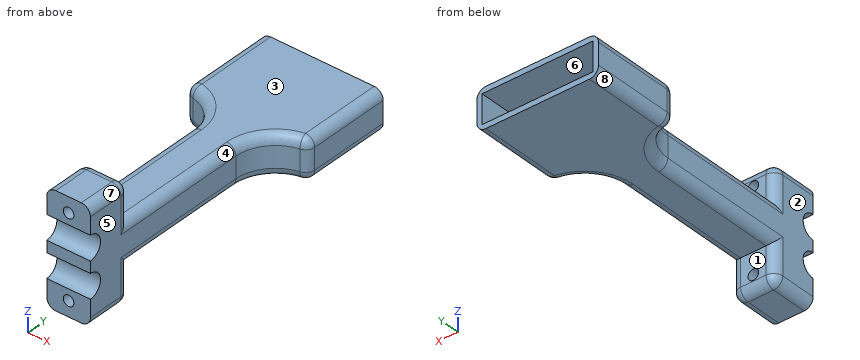
from build123d import *

# Parameters (mm, degrees)
RESSALTO_EXTRUS_O1_DEPTH = 6.5
FILETE1_R                = 3
FILETE2_R                = 3
FILETE3_R                = 13
ESBO_O4_W                = 36.5
ESBO_O4_H                = 9.5
CORTE_EXTRUS_O1_DEPTH    = 25
ESBO_O11_W               = 14.347963754
ESBO_O11_H               = 15
RESSALTO_EXTRUS_O5_DEPTH = 12
ESBO_O17_W               = 14.347963754
ESBO_O17_H               = 15
RESSALTO_EXTRUS_O6_DEPTH = 12
ESBO_O18_R               = 1.75
CORTE_EXTRUS_O5_DEPTH    = 25
ESBO_O19_R               = 3.96875
CORTE_EXTRUS_O6_DEPTH    = 25
FILETE14_R               = 3


with BuildPart() as part:
    # Esboço2 → Ressalto-extrusão1 (new body, symmetric)
    with BuildSketch(Plane.XY):
        Polygon((-20, 50), (20, 50), (20, 20), (7.173981877, 20), (7.173981877, -50), (-7.173981877, -50), (-7.173981877, 20), (-20, 20), align=None)
    extrude(amount=RESSALTO_EXTRUS_O1_DEPTH, both=True)

    # Filete1
    filete1_edges = [part.edges().sort_by_distance(p)[0] for p in [
        (-20, 20, 0),
    ]]
    fillet(filete1_edges, radius=FILETE1_R)

    # Filete2
    filete2_edges = [part.edges().sort_by_distance(p)[0] for p in [
        (20, 20, 0),
    ]]
    fillet(filete2_edges, radius=FILETE2_R)

    # Filete3
    filete3_edges = [part.edges().sort_by_distance(p)[0] for p in [
        (-7.173981877, 20, 0),
        (7.173981877, 20, 0),
    ]]
    fillet(filete3_edges, radius=FILETE3_R)

    # Esboço4 → Corte-extrusão1 (cut)
    with BuildSketch(Plane(origin=(0, 50, 0), x_dir=(1, 0, 0), z_dir=(0, 1, 0))):
        Rectangle(ESBO_O4_W, ESBO_O4_H)
    extrude(amount=-CORTE_EXTRUS_O1_DEPTH, mode=Mode.SUBTRACT)

    # Esboço11 → Ressalto-extrusão5 (add)
    with BuildSketch(Plane.XY.offset(6.5)):
        with Locations((0, -42.5)):
            Rectangle(ESBO_O11_W, ESBO_O11_H)
    extrude(amount=RESSALTO_EXTRUS_O5_DEPTH)

    # Esboço17 → Ressalto-extrusão6 (add)
    with BuildSketch(Plane(origin=(0, 0, -6.5), x_dir=(-1, 0, 0), z_dir=(0, 0, -1))):
        with Locations((0, -42.5)):
            Rectangle(ESBO_O17_W, ESBO_O17_H)
    extrude(amount=RESSALTO_EXTRUS_O6_DEPTH)

    # Esboço18 → Corte-extrusão5 (cut)
    with BuildSketch(Plane.XZ.offset(50)):
        with Locations((0, 13.5)):
            Circle(ESBO_O18_R)
        with Locations((0, -13.5)):
            Circle(ESBO_O18_R)
    extrude(amount=-CORTE_EXTRUS_O5_DEPTH, mode=Mode.SUBTRACT)

    # Esboço19 → Corte-extrusão6 (cut)
    with BuildSketch(Plane.ZY.offset(7.173981877)):
        with Locations((-5.875, -50)):
            Circle(ESBO_O19_R)
        with Locations((5.875, -50)):
            Circle(ESBO_O19_R)
    extrude(amount=-CORTE_EXTRUS_O6_DEPTH, mode=Mode.SUBTRACT)

    # Filete14
    filete14_edges = [part.edges().sort_by_distance(p)[0] for p in [
        (20, 36.5, 6.5),
        (19.322214978, 21.100706027, 6.5),
        (10.111050307, 15.548251086, 6.5),
        (-20, 36.5, 6.5),
        (-19.322214978, 21.100706027, 6.5),
        (-10.111050307, 15.548251086, 6.5),
        (20, 36.5, -6.5),
        (19.322214978, 21.100706027, -6.5),
        (10.111050307, 15.548251086, -6.5),
        (-20, 36.5, -6.5),
        (-19.322214978, 21.100706027, -6.5),
        (-10.111050307, 15.548251086, -6.5),
        (-7.173981877, -42.5, 18.5),
        (-7.173981877, -35, 12.5),
        (0, -35, -18.5),
        (-7.173981877, -35, -12.5),
        (-7.173981877, -42.5, -18.5),
        (7.173981877, -42.5, -18.5),
        (7.173981877, -35, -12.5),
        (7.173981877, -42.5, 18.5),
        (7.173981877, -35, 12.5),
        (0, -35, 18.5),
        (7.173981877, -13.841011399, 6.5),
        (-7.173981877, -13.841011399, 6.5),
        (7.173981877, -13.841011399, -6.5),
        (-7.173981877, -13.841011399, -6.5),
    ]]
    fillet(filete14_edges, radius=FILETE14_R)


solid = part.part
Here's how the part is built. I have some questions about the finished solid (model axes, mm). Face numbers are marked on the shaded views. A direction names the side the tool comes from. Coordinates: 2 decimals unless noted, no trailing zeros. Loops run counter-clockwise (first coordinate to the right, second up) from the corner with the lowest first, then second, coordinate; pieces in that order, holes last.
1. Imagine slicing it at A-A, the plane z = -13.5. Please give me the cut outline in (x, y), and give its area (3 significant figures).
2. For P1, Ø9, axis at x = 1.5, z = -12.5, coming from the +Y side; P2, Ø10, axis at x = -6, y = 19.5, coming from the -Z side; P3, Ø5, axis at x = 11, z = 10.5, coming from the +Y side; P4, Ø1.5, axis at x = -13, z = 1.5, coming from the +Y side, each with a flat end and sliding along its axis, tell me the tip position at first contact or that it passes through.
3. Imagine slicing it at C-C, the plane x = 0. Count the separate pieces of the cut face and the enclosed holes in it, and give its area (3 significant figures).
4. If we mould it in two halves opening along Z, with no side actions, what happens to the marked faces 6, 7 and 8? For each: pulls with the +Z half, pulls with the -Z half, needs draft (parallel to the pull), parting line crosses it, or undercut.
5. Imagine slicing it at D-D, the plane y = -3. Please give me the cut outline in (x, z).
6. Imagine slicing it at B-B, the plane y = 37. Please give me the cut outline in (x, z).
7. For the marked faces 1, 2, 3, 4 and 5, which set-ups out of +Z, -Z, +X, -X, +Y, -Y let a thin tool reach every point of the face, with its end or its side?
8. I need wall thicknesses on L1, parallel to Z at x = 0, y = -42.5; L2, parallel to Z at x = -15, y = 29; L3, parallel to X at y = -11.5, z = 0. Which ranges of each line are inside material? Lowest first, please.
Taken from the geometry:
1. outline: (-7.17, -50) - (-1.75, -50) - (-1.75, -35) - (-4.17, -35) arc R3 ccw to (-7.17, -38) - close; (1.75, -50) - (7.17, -50) - (7.17, -38) arc R3 ccw to (4.17, -35) - (1.75, -35) - close
1. area: 159 mm2
2. P1: stops at y = -35
2. P2: stops at z = -6.5
2. P3: passes through
2. P4: stops at y = 25
3. separate pieces: 3
3. enclosed holes: 0
3. area: 1,260 mm2
4. face 6: undercut
4. face 7: pulls with the +Z half
4. face 8: pulls with the -Z half
5. outline: (-7.17, -3.5) arc R3 ccw to (-4.17, -6.5) - (4.17, -6.5) arc R3 ccw to (7.17, -3.5) - (7.17, 3.5) arc R3 ccw to (4.17, 6.5) - (-4.17, 6.5) arc R3 ccw to (-7.17, 3.5) - close
6. outline: (-20, -3.5) arc R3 ccw to (-17, -6.5) - (17, -6.5) arc R3 ccw to (20, -3.5) - (20, 3.5) arc R3 ccw to (17, 6.5) - (-17, 6.5) arc R3 ccw to (-20, 3.5) - close; hole (-18.25, -4.75) - (18.25, -4.75) - (18.25, 4.75) - (-18.25, 4.75) - close
7. face 1: -Z, +X, -X, +Y
7. face 2: +Z, -Z, -X, -Y
7. face 3: +Z, +X, -X, +Y
7. face 4: +Z, +X
7. face 5: +Z, -Z, +X, -Y
8. L1: z = -18.5 to -15.25, -11.75 to 11.75, 15.25 to 18.5
8. L2: z = -6.5 to -4.75, 4.75 to 6.5
8. L3: x = -7.17 to 7.17
